Autodesk Inventor part; units mm, degrees
ref_plane "YZ Plane" through (0, 0, 0) normal (1, 0, 0) x (0, 1, 0)
ref_plane "XZ Plane" through (0, 0, 0) normal (0, 1, 0) x (-1, 0, 0)
ref_plane "XY Plane" through (0, 0, 0) normal (0, 0, 1) x (1, 0, 0)
sketch "スケッチ1" plane through (0, 0, 0) normal (0, 1, 0) x (-1, 0, 0)
  circle A0 centre (0, 0) radius 5
  circle A1 centre (0, 0) radius 11
  line L0 (0, 0) -> (0, -11)
  line L1 (0, 0) -> (0, 11)
  circle A2 centre (0, 9.5) radius 4.5
  circle A3 centre (0, -9.5) radius 4.5
  circle A4 centre (2.3645, 112.8492) radius 126.872
  circle A5 centre (8.3362, 58.5776) radius 45.2805
  circle A6 centre (2.3645, 112.8492) radius 54.5992
  line L2 (62.25, 31) -> (44.25, 31)
  line L3 (44.25, 31) -> (44.25, 1)
  line L4 (44.25, 1) -> (62.25, 1)
  line L5 (62.25, 1) -> (62.25, 31)
  line L6 (0, 0) -> (13.75, 0)
  line L7 (13.75, 0) -> (13.75, -16.75)
  line L8 (13.75, -16.75) -> (0, -16.75)
  line L9 (0, -16.75) -> (0, 0)
  line L10 (70.25, 35.25) -> (36.25, 35.25)
  line L11 (36.25, 35.25) -> (36.25, -11.25)
  line L12 (36.25, -11.25) -> (70.25, -11.25)
  line L13 (70.25, -11.25) -> (70.25, 35.25)
  line L14 (70.25, 0) -> (36.25, 0)
  line L15 (0, 0) -> (36.25, 0)
  point P0 (62.25, 1)
  point P1 (0.7536, 13.9365)
  point P2 (0, 5)
  point P3 (0, -5)
  point P4 (-0.087, -13.9992)
  dimension "d4" = 253.744
  dimension "d5" = 90.561
  dimension "d0" = 10
  dimension "d1" = 22
  dimension "d2" = 9
  dimension "d3" = 9
  dimension "d7" = 18
  dimension "d8" = 30
  dimension "d9" = 13.75
  dimension "d10" = 16.75
  dimension "d11" = 46.5
  dimension "d12" = 4.25
  dimension "d13" = 8
  dimension "d14" = 34
  dimension "d15" = 11.25
  dimension "d16" = 70.25
extrude "押し出し1" add sketch "スケッチ1" along normal blind 10.25 contours L2 L5 L4 L3
fillet "フィレット1" radius 3 4 edges at (-62.25, 5.125, 31) (-44.25, 5.125, 31) (-62.25, 5.125, 1) (-44.25, 5.125, 1)
sketch "スケッチ5" plane through (0, 10.25, 0) normal (0, 1, 0) x (1, 0, 0)
  line L0 (-59.25, -4) -> (-47.25, -4)
  line L1 (-47.25, -4) -> (-47.25, -28)
  line L2 (-47.25, -28) -> (-59.25, -28)
  line L3 (-59.25, -28) -> (-59.25, -4)
  line L4 (-62.25, -1) -> (-62.25, -28)
  line L5 (-59.25, -31) -> (-47.25, -31)
  point P0 (0, 0)
  point P1 (-62.25, -2.8114)
  dimension "d37" = 3
  dimension "d38" = 3
  dimension "d39" = 12
  dimension "d40" = 24
hole "穴2" at (-59.25, 10.25, 28) at (-47.25, 10.25, 28) at (-47.25, 10.25, 4) at (-59.25, 10.25, 4) direction (0, -1, 0) diameter 2.7 end through all
properties part number "connectpart5"
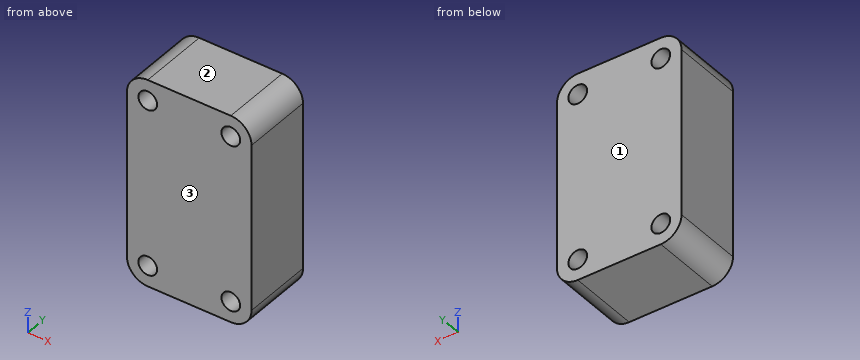
Geometry: final body of the model. Coordinates: model frame, mm. Face numbers are marked on the shaded views. Round coordinates to 2 decimals unless told otherwise and drop trailing zeros. Order: outer loops, then holes, each group sorted by start corner. A loop starts at its lowest first (then second) coordinate and runs counter-clockwise, first axis right, second up.
Q1. Material intervals for probe 1 along X at (y, z) = (5.5, 28); probe 2 along Z at (x, y) = (-59.25, 3.75), sorted ascending.
Result sheet:
probe 1: x = -62.25 to -60.6, -57.9 to -48.6, -45.9 to -44.25
probe 2: z = 1 to 2.65, 5.35 to 26.65, 29.35 to 31
Q2. Mould query, pull axis Y, two halves, no side actions, for the marked faces 1, 2 and 3. Classes: released by +Y, released by -Y, zero draft, split by the parting line, or undercut.
Result sheet:
face 1: released by +Y
face 2: zero draft
face 3: released by -Y
Q3. Section A-A, the plane y = 8. Output: boundary loops of the cut face in (x, z), and give its area (3 significant figures).
Result sheet:
outline: (-62.25, 4) arc R3 ccw to (-59.25, 1) - (-47.25, 1) arc R3 ccw to (-44.25, 4) - (-44.25, 28) arc R3 ccw to (-47.25, 31) - (-59.25, 31) arc R3 ccw to (-62.25, 28) - close; hole circle Ø2.7 at (-59.25, 4); hole circle Ø2.7 at (-59.25, 28); hole circle Ø2.7 at (-47.25, 4); hole circle Ø2.7 at (-47.25, 28)
area: 509 mm2
